Autodesk Inventor part; units mm, degrees
ref_plane "YZ Plane" through (0, 0, 0) normal (1, 0, 0) x (0, 1, 0)
ref_plane "XZ Plane" through (0, 0, 0) normal (0, 1, 0) x (-1, 0, 0)
ref_plane "XY Plane" through (0, 0, 0) normal (0, 0, 1) x (1, 0, 0)
sketch "Sketch1" plane through (0, 0, 0) normal (0, 0, 1) x (1, 0, 0)
  line L0 (-6.35, -3.6662) -> (-6.35, 3.6662)
  line L1 (-6.35, 3.6662) -> (0, 7.3323)
  line L2 (0, 7.3323) -> (6.35, 3.6662)
  line L3 (6.35, 3.6662) -> (6.35, -3.6662)
  line L4 (6.35, -3.6662) -> (0, -7.3323)
  line L5 (0, -7.3323) -> (-6.35, -3.6662)
  point P0 (0, 0)
  point P1 (0, 0)
  dimension "Size" = 12.7
extrude "Extrusion1" add sketch "Sketch1" along normal mid plane 66.294
sketch "Sketch3" plane through (0, 0, 33.147) normal (0, 0, 1) x (1, 0, 0)
  line L0 (-6.35, 3.6662) -> (0, 7.3323) construction
  line L1 (0, 7.3323) -> (6.35, 3.6662) construction
  line L2 (6.35, 3.6662) -> (6.35, -3.6662) construction
  line L3 (6.35, -3.6662) -> (0, -7.3323) construction
  line L4 (0, -7.3323) -> (-6.35, -3.6662) construction
  line L5 (-6.35, -3.6662) -> (-6.35, 3.6662) construction
  point P0 (0, 0)
hole "Hole1" at (0, 0, 33.147) direction (0, 0, -1) diameter 5.1054 end through all
sketch "Sketch4" plane through (0, 0, 33.147) normal (0, 0, 1) x (1, 0, 0)
  circle A0 centre (0, 0) radius 2.5527 construction
  line L0 (-6.35, 3.6662) -> (0, 7.3323) construction
  line L1 (0, 7.3323) -> (6.35, 3.6662) construction
  line L2 (6.35, 3.6662) -> (6.35, -3.6662) construction
  line L3 (6.35, -3.6662) -> (0, -7.3323) construction
  line L4 (0, -7.3323) -> (-6.35, -3.6662) construction
  line L5 (-6.35, -3.6662) -> (-6.35, 3.6662) construction
  circle A1 centre (0, 0) radius 6.8771
  circle A2 centre (0, 0) radius 8.89
  dimension "thunder" = 13.7541
  dimension "d16" = 17.78
extrude "Extrusion3" cut sketch "Sketch4" against normal through all
sketch "Sketch5" plane through (0, 0, 33.147) normal (0, 0, 1) x (1, 0, 0)
  circle A0 centre (0, 0) radius 2.5527
  circle A1 centre (0, 0) radius 6.35
  arc A2 (5.4616, -4.1791) -> (6.35, -2.6403) centre (0, 0) ccw
  line L0 (6.35, -2.6403) -> (6.35, 2.6403)
  arc A3 (6.35, 2.6403) -> (5.4616, 4.1791) centre (0, 0) ccw
  line L1 (5.4616, 4.1791) -> (0.8884, 6.8194)
  arc A4 (0.8884, 6.8194) -> (-0.8884, 6.8194) centre (0, 0) ccw
  line L2 (-0.8884, 6.8194) -> (-5.4616, 4.1791)
  arc A5 (-5.4616, 4.1791) -> (-6.35, 2.6403) centre (0, 0) ccw
  line L3 (-6.35, 2.6403) -> (-6.35, -2.6403)
  arc A6 (-6.35, -2.6403) -> (-5.4616, -4.1791) centre (0, 0) ccw
  line L4 (-5.4616, -4.1791) -> (-0.8884, -6.8194)
  arc A7 (-0.8884, -6.8194) -> (0.8884, -6.8194) centre (0, 0) ccw
  line L5 (0.8884, -6.8194) -> (5.4616, -4.1791)
  circle A8 centre (0, 0) radius 2.5527
  point P0 (3.175, -5.4993)
  point P1 (-3.175, -5.4993)
  point P2 (-6.35, 0)
  point P3 (-3.175, 5.4993)
  point P4 (3.175, 5.4993)
  point P5 (6.35, 0)
  dimension "d21" = 12.7
extrude "Extrusion4" cut sketch "Sketch5" against normal blind 7.9248 contours A0 | L0 A2 L5 A1 | A1 L1 A3 L0 | A1 L2 A4 L1 | L5 A7 L4 A1 | A1 L3 A5 L2 | L4 A6 L3 A1
mirror "Mirror2" about plane through (0, 0, 0) normal (0, 0, 1) of "Extrusion4"
equation "\"bearing\" = 25.4"
properties part number "GP9-007" material "Aluminum 6061"
Model file for the job. Use its own axes, mm. A direction names the side the tool comes from. Give positions to 0.01 mm unless a question says otherwise; leave off trailing zeros. Write each loop counter-clockwise with the first axis right and the second up, starting at its lowest first coordinate (ties: lowest second). Pieces come first, ordered by that corner, then holes. Notation, with made-up numbers: (-4.5, 10.5) -> (14.5, 10.5) arc R31 cw to (14.5, 49.5) -> close; hole circle Ø3 at (4.25, 81.5). An arc over 180 degrees is marked (long way). Use CSV: the item, a comma, the result in double quotes. Start each with the question number.
1) Cut at A-A on x = 0. List the corners of the cut face in (y, z).
2) Tool access for faces 1 (the flat face through (6, -3, 25.222)), 2 (the flat face through (0, 6.5, 25.222)), 3 (the flat face through (-6, 3, 25.222)): list every direction of +Z, -Z, +X, -X, +Y, -Y with a clear straight run to the whole face (end or side of a thin tool).
3) Cut at B-B on y = -2. List the corners of the cut face in (x, z).
4) Drill centre lines: L1, parallel to X at y = 0, z = -8.5; L2, parallel to X at y = -1.25, z = 6; L3, parallel to Y at x = -0.5, z = -16. Where is each one in solid material? Low to high.
5) Cut at D-D on y = 3.5. List the corners of the cut face in (x, z).
6) Pin check, flat tips, straight feed: P1, Ø1.5, axis at x = 1.5, z = 17.5, coming from the +Y side; P2, Ø2, axis at x = 2, z = 6.5, coming from the -Y side; P3, Ø1, axis at y = -4.5, z = -7, coming from the -X side. Stop position of each tip, or through.
7) Cut at C-C on z = -5.5. List the corners of the cut face in (x, y), plus the area to 3 significant figures.
Final values:
1,outline,"(-6.88, -25.22) -> (-6.35, -25.22) -> (-6.35, -33.15) -> (-2.55, -33.15) -> (-2.55, 33.15) -> (-6.35, 33.15) -> (-6.35, 25.22) -> (-6.88, 25.22) -> close; (2.55, -33.15) -> (6.35, -33.15) -> (6.35, -25.22) -> (6.88, -25.22) -> (6.88, 25.22) -> (6.35, 25.22) -> (6.35, 33.15) -> (2.55, 33.15) -> close"
2,face 1,"+Z, +X, -Y"
2,face 2,"+Z, +Y"
2,face 3,"+Z, -X, +Y"
3,outline,"(-6.35, -25.22) -> (-6.03, -25.22) -> (-6.03, -33.15) -> (-1.59, -33.15) -> (-1.59, 33.15) -> (-6.03, 33.15) -> (-6.03, 25.22) -> (-6.35, 25.22) -> close; (1.59, -33.15) -> (6.03, -33.15) -> (6.03, -25.22) -> (6.35, -25.22) -> (6.35, 25.22) -> (6.03, 25.22) -> (6.03, 33.15) -> (1.59, 33.15) -> close"
4,L1,"x = -6.35 to -2.55, 2.55 to 6.35"
4,L2,"x = -6.35 to -2.23, 2.23 to 6.35"
4,L3,"y = -6.86 to -2.5, 2.5 to 6.86"
5,outline,"(-5.92, -25.22) -> (-5.3, -25.22) -> (-5.3, -33.15) -> (5.3, -33.15) -> (5.3, -25.22) -> (5.92, -25.22) -> (5.92, 25.22) -> (5.3, 25.22) -> (5.3, 33.15) -> (-5.3, 33.15) -> (-5.3, 25.22) -> (-5.92, 25.22) -> close"
6,P1,"stops at y = 6.84"
6,P2,"stops at y = -6.75"
6,P3,"stops at x = -5.59"
7,outline,"(-6.35, -2.64) arc R6.88 ccw to (-5.46, -4.18) -> (-0.89, -6.82) arc R6.88 ccw to (0.89, -6.82) -> (5.46, -4.18) arc R6.88 ccw to (6.35, -2.64) -> (6.35, 2.64) arc R6.88 ccw to (5.46, 4.18) -> (0.89, 6.82) arc R6.88 ccw to (-0.89, 6.82) -> (-5.46, 4.18) arc R6.88 ccw to (-6.35, 2.64) -> close; hole circle Ø5.11 at (0, 0)"
7,area,"117 mm2"
